Could you check a few things on this model? Use its own coordinates, in mm. A direction names the side the tool comes from. Coordinates: 2 decimals unless noted, no trailing zeros. Order: outer loops, then holes, each group sorted by start corner. A loop starts at its lowest first (then second) coordinate and runs counter-clockwise, first axis right, second up.
Autodesk Inventor part; units mm, degrees
ref_plane "YZ Plane" through (0, 0, 0) normal (1, 0, 0) x (0, 1, 0)
ref_plane "XZ Plane" through (0, 0, 0) normal (0, 1, 0) x (-1, 0, 0)
ref_plane "XY Plane" through (0, 0, 0) normal (0, 0, 1) x (1, 0, 0)
sketch "Sketch1" plane through (0, 0, 0) normal (0, 1, 0) x (-1, 0, 0)
  line L0 (12.7, 34.1313) -> (-12.7, 34.1313)
  line L1 (-12.7, 34.1313) -> (-12.7, -34.1313)
  line L2 (-12.7, -34.1313) -> (12.7, -34.1313)
  line L3 (12.7, -34.1313) -> (12.7, 34.1313)
  line L4 (12.7, 34.1313) -> (-12.7, -34.1313) construction
  line L5 (-12.7, 34.1313) -> (12.7, -34.1313) construction
  point P0 (0, 0)
  dimension "d0" = 25.4
  dimension "d1" = 68.2625
extrude "Extrusion1" add sketch "Sketch1" along normal blind 5.08
sketch "Sketch2" plane through (0, 5.08, 0) normal (0, 1, 0) x (1, 0, 0)
  line L0 (-5.3975, 11.7221) -> (5.3975, 11.7221)
  line L1 (5.3975, 11.7221) -> (5.3975, -11.7221)
  line L2 (5.3975, -11.7221) -> (-5.3975, -11.7221)
  line L3 (-5.3975, -11.7221) -> (-5.3975, 11.7221)
  line L4 (-5.3975, 11.7221) -> (5.3975, -11.7221) construction
  line L5 (5.3975, 11.7221) -> (-5.3975, -11.7221) construction
  line L6 (-9.2075, 14.2875) -> (9.2075, 14.2875)
  line L7 (9.2075, 14.2875) -> (9.2075, -14.2875)
  line L8 (9.2075, -14.2875) -> (-9.2075, -14.2875)
  line L9 (-9.2075, -14.2875) -> (-9.2075, 14.2875)
  line L10 (-9.2075, 14.2875) -> (9.2075, -14.2875) construction
  line L11 (9.2075, 14.2875) -> (-9.2075, -14.2875) construction
  point P0 (0, 0)
  dimension "d4" = 10.795
  dimension "d5" = 23.4442
  dimension "d6" = 18.415
  dimension "d7" = 28.575
extrude "Extrusion2" add sketch "Sketch2" along normal blind 127
sketch "Sketch4" plane through (0, 132.08, 0) normal (0, 1, 0) x (1, 0, 0)
  point P0 (0, 0)
sketch "Sketch6" plane through (0, 5.08, 0) normal (0, 1, 0) x (1, 0, 0)
  point P0 (0, 0)
sketch "Sketch7" plane through (9.2075, 5.08, -14.2875) normal (0, 0, -1) x (-1, 0, 0)
  line L0 (-3.4925, 0) -> (21.9075, 0)
  circle A0 centre (9.2075, 12.7) radius 3.81
  point P0 (9.2075, -5.08)
  dimension "d13" = 12.7
  dimension "d14" = 7.62
extrude "Extrusion4" cut sketch "Sketch7" against normal blind 5.08
fillet "Fillet1" radius 3.175 4 edges at (0, 5.08, -14.2875) (-9.2075, 5.08, 0) (0, 5.08, 14.2875) (9.2075, 5.08, 0)
properties part number "Bacon1"
Item 1: Thinking about a two-plate mould opening in X: for faces 1 (the face through (0, 5.08, 0)), 2 (the face through (-6, 132.08, 0)), 3 (the face through (-9.208, 69, 0)), which applies, +X half, -X half, draft (parallel to the pull), parting line (faces both ways), or undercut?
Item 2: For pin 1 Ø12 at (x, y) = (-1, 88) entering from -Z; pin 2 Ø5.5 at (x, z) = (1, 5) entering from +Y; pin 3 Ø11.5 at (y, z) = (64.5, 5) entering from -X; pin 4 Ø1 at (y, z) = (25, 15.5) entering from +X, each with a flat end and sliding along its axis, tell me the tip position at first contact or that it passes through.
Item 3: Suppose I cut it at C-C (y = 102.5). List the corners of the cut face in (x, z) for me, and give its area (3 significant figures).
Item 4: Which directions (+Z, -Z, +X, -X, +Y, -Y) give clear straight access to the entire face, cutting with the end or side of a thin tool? Please do faces 4 (the face through (0, 69, 14.288)), 5 (the face through (0, 68, -11.722)), 6 (the face through (0.496, 21.558, -13.023)).
Item 5: I need wall thicknesses on line 1 (Y direction, x = 0, z = -12.25); line 2 (Z direction, x = 3.5, y = 15.5); line 3 (X direction, y = 72, z = -1). Which ranges of each line are inside material? Lowest first, please.
Geometry results:
1. face 1: undercut
1. face 2: draft
1. face 3: -X half
2. pin 1: stops at z = -14.29
2. pin 2: stops at y = 5.08
2. pin 3: stops at x = -9.21
2. pin 4: passes through
3. outline: (-9.21, -14.29) - (9.21, -14.29) - (9.21, 14.29) - (-9.21, 14.29) - close; hole (-5.4, -11.72) - (5.4, -11.72) - (5.4, 11.72) - (-5.4, 11.72) - close
3. area: 273 mm2
4. face 4: +Z, +X, -X, +Y
4. face 5: +Y
4. face 6: -Z
5. line 1: y = 0 to 13.97, 21.59 to 132.08
5. line 2: z = -14.29 to -11.72, 11.72 to 14.29
5. line 3: x = -9.21 to -5.4, 5.4 to 9.21
